Geometry check sheet. Reference: the model listing, model coordinates, mm. A direction names the side the tool comes from. Coordinates: 2 decimals unless noted, no trailing zeros. Write each loop counter-clockwise with the first axis right and the second up, starting at its lowest first coordinate (ties: lowest second). Pieces come first, ordered by that corner, then holes.
from build123d import *

# Parameters (mm, degrees)
F1_DEPTH      = 5
F3_DEPTH      = 5
F3_DEPTH_BACK = 5
F4_R          = 2.5
F5_DEPTH      = 5.001


with BuildPart() as f1:
    # F0 (on Front) → F1 (new body)
    with BuildSketch(Plane.XZ):
        with BuildLine():
            Line((0, 9.13175), (0, 7.5))
            ThreePointArc((0, 7.5), (-6.835784, -3.085784), (5.625, -4.960784))
            Line((5.625, -4.960784), (10, 0))
            Line((10, 0), (10, 10))
            Line((10, 10), (3.75, 25))
            Line((3.75, 25), (1.25, 25))
            Line((1.25, 25), (1.25, 10))
            Line((1.25, 10), (0, 9.13175))
        make_face()
    extrude(amount=F1_DEPTH)

    # F2 (on face) → F3 (join, two sides)
    with BuildSketch(Plane.XZ.offset(5)) as f3_sk:
        with BuildLine():
            Line((3.75, 25), (1.25, 25))
            Line((1.25, 25), (1.25, 23.75))
            Line((1.25, 23.75), (-1.25, 22.5))
            Line((-1.25, 22.5), (1.25, 21.25))
            Line((1.25, 21.25), (-1.25, 20))
            Line((-1.25, 20), (1.25, 18.75))
            Line((1.25, 18.75), (-1.25, 17.5))
            Line((-1.25, 17.5), (1.25, 16.25))
            Line((1.25, 16.25), (-1.25, 15))
            Line((-1.25, 15), (1.25, 13.75))
            Line((1.25, 13.75), (-1.25, 12.5))
            Line((-1.25, 12.5), (1.25, 11.25))
            Line((1.25, 11.25), (-1.25, 10))
            Line((-1.25, 10), (0, 9.375))
            Line((0, 9.375), (0, 9.13175))
            Line((0, 9.13175), (0, 8.5))
            ThreePointArc((0, 8.5), (6.667708, 5.27178), (8.270751, -1.960784))
            Line((8.270751, -1.960784), (10, 0))
            Line((10, 0), (10, 10))
            Line((10, 10), (3.75, 25))
        make_face()
        Polygon((1.25, 23.75), (1.25, 25), (-1.25, 25), align=None)
    extrude(amount=F3_DEPTH)
    extrude(f3_sk.sketch, amount=-F3_DEPTH_BACK)

    # F4 (on face) → F5 (cut, through all)
    with BuildSketch(Plane.XZ.offset(5)):
        Circle(F4_R)
    extrude(amount=-F5_DEPTH, mode=Mode.SUBTRACT)


with BuildPart() as f6_1:
    # F6: copy of F1
    add(f1.part)


with BuildPart() as f8_1:
    # F8: copy of F1
    add(f1.part.moved(Location((20, 0, 0))))


with BuildPart() as f10_1:
    # F10: copy of F1
    add(f1.part)


solid = f1.part
1. Sectioned sample at C-C, the plane x = -1.75. Record the boundary of the cut face in (y, z).
Computed values:
outline: (-5, -7.29) - (0, -7.29) - (0, -1.79) - (-5, -1.79) - close; (-5, 1.79) - (0, 1.79) - (0, 7.29) - (-5, 7.29) - close
2. Sectioned sample at A-A, the plane y = -0.75. Record the boundary of the cut face in (x, z) (3 decimals), and give its area (3 significant figures).
Computed values:
outline: (-1.25, 10) - (0, 9.375) - (0, 7.5) arc R7.5 ccw (long way) to (5.625, -4.961) - (10, 0) - (10, 10) - (3.75, 25) - (-1.25, 25) - (1.25, 23.75) - (-1.25, 22.5) - (1.25, 21.25) - (-1.25, 20) - (1.25, 18.75) - (-1.25, 17.5) - (1.25, 16.25) - (-1.25, 15) - (1.25, 13.75) - (-1.25, 12.5) - (1.25, 11.25) - close; hole circle Ø5 at (0, 0)
area: 321 mm2
3. Thickness scan on line 1 along Y through (x, z) = (4.5, 5.5); line 2 along X through (y, z) = (-2, -2); line 3 along Z through (x, y) = (-1.75, -3.25). Record the ranges inside material, lowest first.
Computed values:
line 1: y = -5 to 0
line 2: x = -7.23 to -1.5, 1.5 to 8.24
line 3: z = -7.29 to -1.79, 1.79 to 7.29
4. Gauge pin test, flat ends, axial feed: pin 1 Ø2 at (y, z) = (-7, -3) entering from -X; pin 2 Ø1 at (y, z) = (-9, 0.5) entering from -X; pin 3 Ø1 at (x, y) = (5.5, -4.5) entering from -Z; pin 4 Ø0.9 at (y, z) = (-3.5, 8) entering from -X. Record the tip position at first contact, or that the pin passes through.
Computed values:
pin 1: passes through
pin 2: stops at x = 8.44
pin 3: stops at z = -5.59
pin 4: stops at x = 0
5. Access from +Z, -Z, +X, -X, +Y, -Y to the whole of each face (thin tool, end or side, straight path). Record for faces 1 (the cylindrical face through (6.601, -7.465, 5.356)), 2 (the flat face through (1, -5, 25)), 3 (the flat face through (-0.017, -5.07, 21.884)).
Computed values:
face 1: -X, -Y
face 2: +Z, +X, -X, +Y, -Y
face 3: -X, +Y, -Y
6. Sectioned sample at B-B, the plane z = 0.5. Record the boundary of the cut face in (x, y).
Computed values:
outline: (-7.48, -5) - (-2.45, -5) - (-2.45, 0) - (-7.48, 0) - close; (2.45, -5) - (8.49, -5) - (8.49, -10) - (10, -10) - (10, 0) - (2.45, 0) - close
7. Sectioned sample at D-D, the plane y = -7.75. Record the boundary of the cut face in (x, z) (3 decimals), and give its area (3 significant figures).
Computed values:
outline: (-1.25, 10) - (0, 9.375) - (0, 8.5) arc R8.5 cw to (8.271, -1.961) - (10, 0) - (10, 10) - (3.75, 25) - (-1.25, 25) - (1.25, 23.75) - (-1.25, 22.5) - (1.25, 21.25) - (-1.25, 20) - (1.25, 18.75) - (-1.25, 17.5) - (1.25, 16.25) - (-1.25, 15) - (1.25, 13.75) - (-1.25, 12.5) - (1.25, 11.25) - close
area: 148 mm2
8. Draft check along Z on faces 4 (the flat face through (3, 0, 5)), 5 (the flat face through (0.017, -5.07, 15.634)), 6 (the flat face through (6.919, -4.93, 17.395)). Enter one of: released by +Z, released by -Z, zero draft, split by the parting line, or undercut.
Computed values:
face 4: zero draft
face 5: undercut
face 6: released by +Z
